Autodesk Inventor part; units mm, degrees
ref_plane "YZ Plane" through (0, 0, 0) normal (1, 0, 0) x (0, 1, 0)
ref_plane "XZ Plane" through (0, 0, 0) normal (0, 1, 0) x (-1, 0, 0)
ref_plane "XY Plane" through (0, 0, 0) normal (0, 0, 1) x (1, 0, 0)
sketch "Sketch1" plane through (0, 0, 0) normal (1, 0, 0) x (0, 1, 0)
  line L0 (0, 0) -> (2.5, 0)
  line L1 (0, 0) -> (4, 0)
  line L2 (2.5, 0) -> (2.5, -7)
  line L3 (2.5, -7) -> (0, -7)
  line L4 (0, -7) -> (20, -7)
  line L5 (4, 0) -> (4, -7)
  line L6 (2.5, -7) -> (2.5, -41)
  line L7 (20, -7) -> (20, -11)
  line L8 (20, -11) -> (2.5, -11)
  line L9 (20, -7) -> (22.5, -7)
  line L10 (22.5, -7) -> (22.5, -11)
  line L11 (22.5, -11) -> (20, -11)
  line L12 (20, -11) -> (20, -7)
  line L13 (20, -7) -> (20, -11)
  line L14 (4, 0) -> (2.5, 0)
  line L15 (2.5, 0) -> (2.5, -11)
  line L16 (2.5, -11) -> (4, -11)
  line L17 (4, -11) -> (4, 0)
  line L18 (2.5, -11) -> (22.5, -11)
  line L19 (22.5, -11) -> (22.5, -7)
  line L20 (22.5, -7) -> (2.5, -7)
  line L21 (2.5, -7) -> (2.5, -11)
  line L22 (2.5, -11) -> (6.5, -11)
  line L23 (0, -7) -> (0, -105.9451)
  line L24 (2.5, -41) -> (25, -41)
  line L25 (0, -82) -> (2.5, -82)
  line L26 (0, -82) -> (4, -82)
  line L27 (2.5, -82) -> (2.5, -75)
  line L28 (2.5, -75) -> (0, -75)
  line L29 (0, -75) -> (20, -75)
  line L30 (4, -82) -> (4, -75)
  line L31 (20, -75) -> (20, -71)
  line L32 (20, -71) -> (2.5, -71)
  line L33 (20, -75) -> (22.5, -75)
  line L34 (22.5, -75) -> (22.5, -71)
  line L35 (22.5, -71) -> (20, -71)
  line L36 (20, -71) -> (20, -75)
  line L37 (20, -75) -> (20, -71)
  line L38 (4, -82) -> (2.5, -82)
  line L39 (2.5, -82) -> (2.5, -71)
  line L40 (2.5, -71) -> (4, -71)
  line L41 (4, -71) -> (4, -82)
  line L42 (2.5, -71) -> (22.5, -71)
  line L43 (22.5, -71) -> (22.5, -75)
  line L44 (22.5, -75) -> (2.5, -75)
  line L45 (2.5, -75) -> (2.5, -71)
  line L46 (2.5, -71) -> (6.5, -71)
  line L47 (2.5, -11) -> (6.5, -11)
  line L48 (6.5, -11) -> (6.5, -71)
  line L49 (6.5, -71) -> (2.5, -71)
  line L50 (2.5, -71) -> (2.5, -11)
  line L51 (6.5, -11) -> (9.5, -11)
  line L52 (9.5, -11) -> (9.5, -14)
  line L53 (9.5, -14) -> (6.5, -14)
  line L54 (6.5, -14) -> (6.5, -11)
  line L55 (6.5, -71) -> (9.5, -71)
  line L56 (9.5, -71) -> (9.5, -68)
  line L57 (9.5, -68) -> (6.5, -68)
  line L58 (6.5, -68) -> (6.5, -71)
  dimension "d1" = 2.5
  dimension "d2" = 4
  dimension "d3" = 7
  dimension "d4" = 20
  dimension "d5" = 34
  dimension "d9" = 4
  dimension "d12" = 2.5
  dimension "d13" = 4
  dimension "d55" = 22.5
  dimension "d56" = 4
  dimension "d80" = 3
  dimension "d81" = 3
  dimension "d82" = 3
  dimension "d83" = 3
revolve "Revolution2" add sketch "Sketch1" angle 360 about axis through (0, 0, -7) along (0, 0, -1) contours L1 L5 L4 L2 | L4 L17 L8 L6 | L4 L7 L8 L17 | L8 L48 L24 L6 | L9 L10 L11 L7 | L24 L48 L32 L50 | L8 L52 L53 L48 | L29 L30 L26 L27 | L39 L32 L41 L29 | L41 L32 L31 L29 | L57 L56 L32 L48 | L31 L35 L34 L33
sketch "Sketch6" plane through (0, 0, 0) normal (0, 1, 0) x (-1, 0, 0)
  line L0 (-2.5, -82) -> (2.5, -82)
  line L1 (0, -82) -> (0, -62)
  line L2 (0, -82) -> (20, -82) construction
  line L3 (0, -65) -> (15, -65) construction
  line L4 (0, -59) -> (15, -59) construction
  line L5 (10.6066, -48.3934) -> (10.6066, -54.3934)
  line L6 (0, -65) -> (0, -59)
  line L7 (0, -62) -> (0, -59.5)
  line L8 (0, -59.5) -> (10.6066, -48.8934)
  line L9 (10.6066, -48.8934) -> (10.6066, -53.8934)
  line L10 (10.6066, -53.8934) -> (0, -64.5)
  line L11 (0, -59.5) -> (0, -64.5)
  point P0 (0, 0)
  dimension "d64" = 20
  dimension "d65" = 90
  dimension "d69" = 15
  dimension "d71" = 15
  dimension "d75" = 2.5
  dimension "d76" = 5
extrude "Extrusion6" cut sketch "Sketch6" along normal mid plane 5
sketch "Sketch7" plane through (0, 0, 0) normal (0, 0, 1) x (1, 0, 0)
  arc A0 (-1.9966, -1.5104) -> (-1.9966, 1.4896) centre (0.0034, -0.0104) ccw
  line L0 (-1.9966, -0.0104) -> (-1.9966, 1.4896)
  line L1 (-1.9966, -0.0104) -> (-1.9966, -1.5104)
  line L2 (-1.9966, 1.4896) -> (-1.9966, -2.007)
  line L3 (-1.9966, -2.007) -> (-3.9862, -2.007)
  line L4 (-3.9862, -2.007) -> (-3.9862, 1.4896)
  line L5 (-3.9862, 1.4896) -> (-1.9966, 1.4896)
  line L6 (-1.9966, -1.5104) -> (-3.2272, -1.5104)
  line L7 (-3.2272, -1.5104) -> (-3.2272, 1.4896)
  line L8 (-3.2272, 1.4896) -> (-1.9966, 1.4896)
  line L9 (-1.9966, 1.4896) -> (-1.9966, -1.5104)
  point P0 (0, 0)
  point P1 (0, 0)
  dimension "d77" = 5
extrude "Extrusion7" add sketch "Sketch7" against normal blind 26 contours L6 L7 L5 L0 L1
properties part number "Spool_revB"
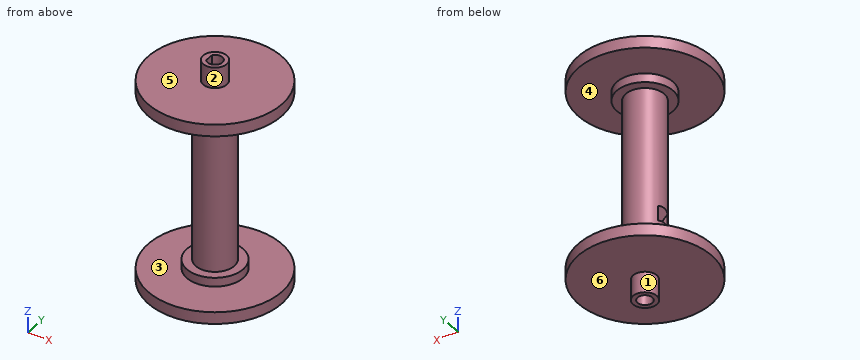
The listing builds one solid part. Answer for the finished solid, in the listing's coordinates (mm). Face numbers are marked on the shaded views. A direction names the side the tool comes from. Give positions to 0.01 mm unless a question says otherwise; leave off trailing zeros. Loops run counter-clockwise (first coordinate to the right, second up) from the corner with the lowest first, then second, coordinate; pieces in that order, holes last. Notation, with made-up numbers: M 77.5,65.5 L 118.5,65.5 A20 cw 118.5,83.5 Z; hole C -21.5,1.25 d6. An arc over 180 degrees is marked long. One line per item, written item: value.
1. Each of these flat-tipped pins is pushed along its axis until it touches: P1, Ø1, axis at x = -14, y = -10.5, coming from the -Z side; P2, Ø3.5, axis at y = 0, z = -7.5, coming from the +X side; P3, Ø1.5, axis at y = -6, z = -52.5, coming from the -X side. Where does it stop, or does it pass through?
Found:
P1: z = -75
P2: x = 22.5
P3: x = -3.83
2. Section D-D on x = -14 is taken. Determine the outline of the cut face in (y, z), plus the area to 3 significant figures.
Found:
outline: M -17.61,-75 L 17.61,-75 L 17.61,-71 L -17.61,-71 Z; M -17.61,-11 L 17.61,-11 L 17.61,-7 L -17.61,-7 Z
area: 282 mm^2
3. Section C-C on y = 0 is taken. State how many separate pieces and enclosed holes the cut face has, plus the area to 3 significant figures.
Found:
separate pieces: 3
enclosed holes: 0
area: 871 mm^2
4. Section B-B on z = -51 is taken. Determine the outline of the cut face in (x, y).
Found:
outline: C 0,0 d13; hole C 0,0 d5
5. For the marked faces 1, 2 and 3, determine the directions among +Z, -Z, +X, -X, +Y, -Y from which every point of the face is accessible in a straight line to the end or side of a thin tool.
Found:
face 1: -Z
face 2: +Z
face 3: none
6. Section A-A on x = 13.5 is taken. Determine the outline of the cut face in (y, z).
Found:
outline: M -18,-75 L 18,-75 L 18,-71 L -18,-71 Z; M -18,-11 L 18,-11 L 18,-7 L -18,-7 Z
7. For a pull along Z with two mould halves and no side action, classify the marked faces 4, 5 and 6 as pulls with the +Z half, pulls with the -Z half, needs draft (parallel to the pull), parting line crosses it, or undercut.
Found:
face 4: undercut
face 5: pulls with the +Z half
face 6: pulls with the -Z half
8. Find the intervals of material crossed by probe 1 along X at (y, z) = (0, -39); probe 2 along Z at (x, y) = (14.5, -11); probe 3 along X at (y, z) = (0, -20), in increasing order.
Found:
probe 1: -6.5 to -2.5, 2.5 to 6.5
probe 2: -75 to -71, -11 to -7
probe 3: -6.5 to -2, 2.5 to 6.5
